Work out the finished part from the listing and answer in its coordinate system (mm). Give positions to 0.01 mm unless a question says otherwise; leave off trailing zeros. Loops run counter-clockwise (first coordinate to the right, second up) from the corner with the lowest first, then second, coordinate; pieces in that order, holes last. Notation, with made-up numbers: (54, 40.25) - (58, 40.25) arc R16 ccw to (58, 68.25) - close; hole circle Ø9 at (4.5, 25). An arc over 180 degrees is marked (long way). One line per item, written item: value.
from build123d import *

# Parameters (mm, degrees)
SKETCH1_W           = 80
SKETCH1_H           = 40
BOSS_EXTRUDE1_DEPTH = 20
BOSS_EXTRUDE2_START = 40
BOSS_EXTRUDE2_DEPTH = 25
FILLET1_R           = 15


with BuildPart() as part:
    # Sketch1 → Boss-Extrude1 (new, symmetric)
    with BuildSketch(Plane(origin=(0, 0, 0), x_dir=(1, 0, 0), z_dir=(0, 1, 0))):
        Rectangle(SKETCH1_W, SKETCH1_H)
    extrude(amount=BOSS_EXTRUDE1_DEPTH, both=True)

    # Sketch4 → Boss-Extrude2 (add)
    with BuildSketch(Plane(origin=(0, 0, 0), x_dir=(0, 0, -1), z_dir=(1, 0, 0)).offset(BOSS_EXTRUDE2_START)):
        with BuildLine():
            ThreePointArc((2, 0), (1, 1.732050808), (-1, 1.732050808))
            Line((-1, 1.732050808), (-1, -1.732050808))
            ThreePointArc((-1, -1.732050808), (1, -1.732050808), (2, 0))
        make_face()
    extrude(amount=BOSS_EXTRUDE2_DEPTH)

    # Fillet1
    fillet1_edges = [part.edges().sort_by_distance(p)[0] for p in [
        (0, 20, 20),
        (0, 20, -20),
    ]]
    fillet(fillet1_edges, radius=FILLET1_R)


solid = part.part
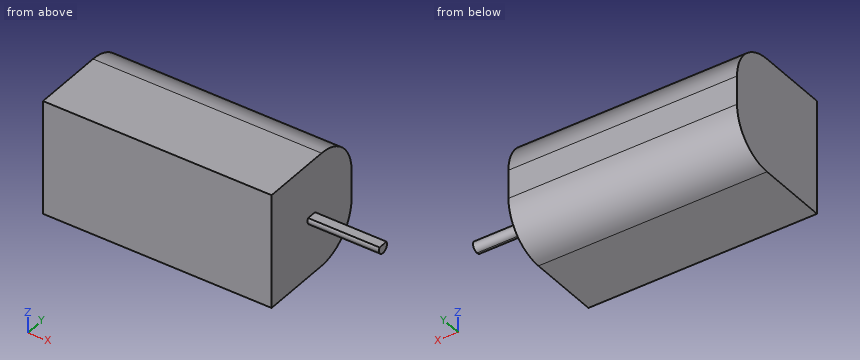
1. Section D-D (x = 54) is taken. Write down the section's boundary in (y, z).
Output:
outline: (-1.73, 1) arc R2 ccw (long way) to (1.73, 1) - close
2. Flat-ended cylindrical pins translate along their axes: pin 1 Ø4 at (x, y) = (51.5, -1) entering from +Z; pin 2 Ø6 at (x, z) = (18, 8.5) entering from +Y. Find the tip coordinate at first contact, or state that the pin passes through.
Output:
pin 1: stops at z = 1
pin 2: stops at y = 19.99
3. Section B-B (z = 2.5) is taken. Write down the section's boundary in (x, y), and give its area (3 significant figures).
Output:
outline: (-40, -20) - (40, -20) - (40, 20) - (-40, 20) - close
area: 3,200 mm²
4. Section C-C (y = 14) is taken. Write down the section's boundary in (x, z), and give its area (3 significant figures).
Output:
outline: (-40, -17) - (40, -17) - (40, 17) - (-40, 17) - close
area: 2,720 mm²
5. Section A-A (x = 9) is taken. Write down the section's boundary in (y, z).
Output:
outline: (-20, -20) - (5, -20) arc R15 ccw to (20, -5) - (20, 5) arc R15 ccw to (5, 20) - (-20, 20) - close
6. Find the intervals of material crossed by line 1 along X through (y, z) = (-4.5, 8); line 2 along Y through (x, z) = (-2, 17); line 3 along Y through (x, z) = (-17, 15), in increasing order.
Output:
line 1: x = -40 to 40
line 2: y = -20 to 14
line 3: y = -20 to 16.18
